Can you work these out from the model? Positions are in its coordinate system, mm. A direction names the side the tool comes from. Give positions to 0.01 mm unless a question says otherwise; leave off trailing zeros. Write each loop counter-clockwise with the first axis right and the second up, starting at its lowest first coordinate (ties: lowest second). Pieces come first, ordered by that corner, then holes. Notation, with made-up numbers: (-17, 53.5) -> (38, 53.5) arc R22 ccw to (38, 86.5) -> close; hole circle Ø3 at (65.5, 45). An arc over 180 degrees is marked (long way). Answer as CSV lines item,"result". Start each with the question number.
1. If we section it at B-B on z = 0: Write out the boundary of the cut face in (x, y).
2. On a 3-axis mill with a long thin cutter (end or side, diameter ignored), from which of +Z, -Z, +X, -X, +Y, -Y can I reach the whole of each face in a straight line? I mean faces 1 (the face through (-14.985, 16.233, 0.66)), 2 (the face through (-11.18, 15, -7.85)). Say none if no direction works.
3. I'm going to push flat-ended pins straight in: P1, Ø2, axis at y = 3, z = 6.5, coming from the +X side; P2, Ø10, axis at x = 3, y = 4, coming from the -Z side; P3, Ø3, axis at y = 1, z = -5.5, coming from the -X side; P4, Ø4, axis at y = 10.5, z = 2, coming from the -X side. Where does each tip first touch, or does it pass through?
4. I need wall thicknesses on line 1 (Y direction, x = -12.5, z = -6); line 2 (X direction, y = 1.5, z = 0). Which ranges of each line are inside material? Lowest first, please. Write a range as [from, to].
5. If we mould it in two halves opening along Z, with no side actions, what happens to faces 3 (the face through (-0.54, 7.36, -2.44)), 4 (the face through (-2.93, 7.4, -13.18)), 5 (the face through (-11.18, 0, -7.85))? For each: pulls with the +Z half, pulls with the -Z half, needs draft (parallel to the pull), parting line crosses it, or undercut.
6. If we section it at A-A on x = 0: Write out the boundary of the cut face in (y, z).
7. If we section it at C-C on y = -1: Write out the boundary of the cut face in (x, z), plus the area to 3 significant figures.
8. If we section it at D-D on z = -3.25: Write out the boundary of the cut face in (x, y).
Autodesk Fusion 360 part; units mm, degrees
sketch "Sketch1" plane through (0, 0, 0) normal (0, 1, 0) x (1, 0, 0)
  circle A0 centre (0, 0) radius 2.5
  circle A1 centre (0, 0) radius 13.5
  circle A2 centre (0, 0) radius 15
  dimension "d1" = 5
  dimension "d2" = 27
extrude "Extrude1" add sketch "Sketch1" against normal blind 2.5 contours A1 | A2
extrude "Extrude2" add sketch "Sketch1" along normal blind 15 contours A1
extrude "Extrude3" add sketch "Sketch1" along normal blind 2.5 from surface at 15 contours A1 | A2
Computed values:
1,outline,"(-15, -2.5) -> (-2.5, -2.5) -> (-2.5, 17.5) -> (-15, 17.5) -> (-15, 15) -> (-13.5, 15) -> (-13.5, 0) -> (-15, 0) -> close; (2.5, -2.5) -> (15, -2.5) -> (15, 0) -> (13.5, 0) -> (13.5, 15) -> (15, 15) -> (15, 17.5) -> (2.5, 17.5) -> close"
2,face 1,"+Y, -Y"
2,face 2,"none"
3,P1,"stops at x = 12.33"
3,P2,"stops at z = -15"
3,P3,"stops at x = -14.35"
3,P4,"stops at x = -13.5"
4,line 1,"y = [-2.5, 0], [15, 17.5]"
4,line 2,"x = [-13.5, -2.5], [2.5, 13.5]"
5,face 3,"undercut"
5,face 4,"parting line crosses it"
5,face 5,"needs draft"
6,outline,"(-2.5, -15) -> (0, -15) -> (0, -13.5) -> (15, -13.5) -> (15, -15) -> (17.5, -15) -> (17.5, -2.5) -> (-2.5, -2.5) -> close; (-2.5, 2.5) -> (17.5, 2.5) -> (17.5, 15) -> (15, 15) -> (15, 13.5) -> (0, 13.5) -> (0, 15) -> (-2.5, 15) -> close"
7,outline,"circle Ø30 at (0, 0); hole circle Ø5 at (0, 0)"
7,area,"687 mm2"
8,outline,"(-14.64, -2.5) -> (14.64, -2.5) -> (14.64, 0) -> (13.1, 0) -> (13.1, 15) -> (14.64, 15) -> (14.64, 17.5) -> (-14.64, 17.5) -> (-14.64, 15) -> (-13.1, 15) -> (-13.1, 0) -> (-14.64, 0) -> close"
